Source: CAD feature listing. Evaluate the final solid. Frame: model axes, mm. Round coordinates to 2 decimals unless told otherwise and drop trailing zeros. Write each loop counter-clockwise with the first axis right and the second up, starting at its lowest first coordinate (ties: lowest second). Pieces come first, ordered by that corner, then holes. Notation, with made-up numbers: M 1,79.5 L 25,79.5 A20 ccw 25,112.5 Z; hole C 6.5,45 d6. An arc over 180 degrees is marked long. Answer in a Markdown table with one row per item.
from build123d import *

# Parameters (mm, degrees)
SKETCH1_R           = 2.55
SKETCH1_R_2         = 3.4
BOSS_EXTRUDE1_DEPTH = 120


with BuildPart() as part:
    # Sketch1 → Boss-Extrude1 (new body)
    with BuildSketch(Plane.XY):
        with BuildLine():
            Line((-13, -15), (-4, -15))
            Line((-4, -15), (-4, -13))
            Line((-4, -13), (-8.25, -13))
            Line((-8.25, -13), (-8.25, -9.664213562))
            Line((-8.25, -9.664213562), (-4.585786438, -6))
            Line((-4.585786438, -6), (4.585786438, -6))
            Line((4.585786438, -6), (8.25, -9.664213562))
            Line((8.25, -9.664213562), (8.25, -13))
            Line((8.25, -13), (4, -13))
            Line((4, -13), (4, -15))
            Line((4, -15), (13, -15))
            ThreePointArc((13, -15), (14.414213562, -14.414213562), (15, -13))
            Line((15, -13), (15, -4))
            Line((15, -4), (13, -4))
            Line((13, -4), (13, -8.25))
            Line((13, -8.25), (9.664213562, -8.25))
            Line((9.664213562, -8.25), (6, -4.585786438))
            Line((6, -4.585786438), (6, 4.585786438))
            Line((6, 4.585786438), (9.664213562, 8.25))
            Line((9.664213562, 8.25), (13, 8.25))
            Line((13, 8.25), (13, 4))
            Line((13, 4), (15, 4))
            Line((15, 4), (15, 13))
            ThreePointArc((15, 13), (14.414213562, 14.414213562), (13, 15))
            Line((13, 15), (4, 15))
            Line((4, 15), (4, 13))
            Line((4, 13), (8.25, 13))
            Line((8.25, 13), (8.25, 9.664213562))
            Line((8.25, 9.664213562), (4.585786438, 6))
            Line((4.585786438, 6), (-4.585786438, 6))
            Line((-4.585786438, 6), (-8.25, 9.664213562))
            Line((-8.25, 9.664213562), (-8.25, 13))
            Line((-8.25, 13), (-4, 13))
            Line((-4, 13), (-4, 15))
            Line((-4, 15), (-13, 15))
            ThreePointArc((-13, 15), (-14.414213562, 14.414213562), (-15, 13))
            Line((-15, 13), (-15, 4))
            Line((-15, 4), (-13, 4))
            Line((-13, 4), (-13, 8.25))
            Line((-13, 8.25), (-9.664213562, 8.25))
            Line((-9.664213562, 8.25), (-6, 4.585786438))
            Line((-6, 4.585786438), (-6, -4.585786438))
            Line((-6, -4.585786438), (-9.664213562, -8.25))
            Line((-9.664213562, -8.25), (-13, -8.25))
            Line((-13, -8.25), (-13, -4))
            Line((-13, -4), (-15, -4))
            Line((-15, -4), (-15, -13))
            ThreePointArc((-15, -13), (-14.414213562, -14.414213562), (-13, -15))
        make_face()
        with Locations(Location((-11.6, 11.6, 0), (0, 0, 180))):  # turned: the seam where the file's is
            Circle(SKETCH1_R, mode=Mode.SUBTRACT)
        with Locations(Location((0, 0, 0), (0, 0, 180))):  # turned: the seam where the file's is
            Circle(SKETCH1_R_2, mode=Mode.SUBTRACT)
        with Locations(Location((-11.6, -11.6, 0), (0, 0, 180))):  # turned: the seam where the file's is
            Circle(SKETCH1_R, mode=Mode.SUBTRACT)
        with Locations(Location((11.6, -11.6, 0), (0, 0, 180))):  # turned: the seam where the file's is
            Circle(SKETCH1_R, mode=Mode.SUBTRACT)
        with Locations(Location((11.6, 11.6, 0), (0, 0, 180))):  # turned: the seam where the file's is
            Circle(SKETCH1_R, mode=Mode.SUBTRACT)
    extrude(amount=BOSS_EXTRUDE1_DEPTH)


solid = part.part
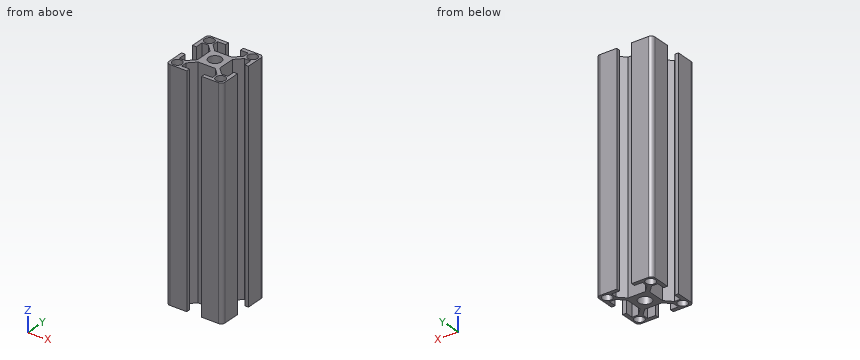
Q1. Contact query for flat-ended pins moving along their axis: pin 1 Ø0.6 at (x, z) = (14, 85) entering from +Y; pin 2 Ø1.6 at (y, z) = (14, 71) entering from +X. Output: stop coordinate, or through.
Solutions:
| item | result |
|---|---|
| pin 1 | stops at y = 14.87 |
| pin 2 | stops at x = 14.99 |
Q2. Section A-A (x = -11.6). Return loops of the section in (y, z), and give its area (3 significant figures).
Solutions:
| item | result |
|---|---|
| outline | M -15,0 L -14.15,0 L -14.15,120 L -15,120 Z; M -9.05,0 L -8.25,0 L -8.25,120 L -9.05,120 Z; M 8.25,0 L 9.05,0 L 9.05,120 L 8.25,120 Z; M 14.15,0 L 15,0 L 15,120 L 14.15,120 Z |
| area | 396 mm2 |
Q3. Material intervals for probe 1 along Y at (x, z) = (11.25, 53.5); probe 2 along X at (y, z) = (11.6, 45); probe 3 along Y at (x, z) = (-5.75, 67), sorted ascending.
Solutions:
| item | result |
|---|---|
| probe 1 | y = -15 to -14.13, -9.07 to -8.25, 8.25 to 9.07, 14.13 to 15 |
| probe 2 | x = -15 to -14.15, -9.05 to -8.25, 8.25 to 9.05, 14.15 to 15 |
| probe 3 | y = -15 to -13, -7.16 to 7.16, 13 to 15 |
Q4. Section B-B (y = 0). Return loops of the section in (x, z).
Solutions:
| item | result |
|---|---|
| outline | M -6,0 L -3.4,0 L -3.4,120 L -6,120 Z; M 3.4,0 L 6,0 L 6,120 L 3.4,120 Z |
